For this review, take the finished solid that the model builds, in its own axes (mm). A direction names the side the tool comes from. Coordinates: 2 decimals unless noted, no trailing zeros. Loops run counter-clockwise (first coordinate to the right, second up) from the corner with the lowest first, then second, coordinate; pieces in that order, holes last. Notation, with made-up numbers: (20, 0.5) - (47, 0.5) arc R21 ccw to (47, 13.5) - close; hole circle Ø5 at (89, 19). An arc over 180 degrees is marked (long way). Use one line per item in the form item = value. Start each with the question number.
1. To check wall thickness, follow probe 1 along Y at (x, z) = (0, 12); probe 2 along X at (y, z) = (-37, 14); probe 3 along X at (y, z) = (9, 3.5). State the ranges of each line that lie inside material, in increasing order.
2. For pin 1 Ø1.2 at (x, y) = (-40, 1) entering from +Z; pin 2 Ø2.5 at (x, y) = (2.5, 40.5) entering from +Z; pin 3 Ø2 at (x, z) = (11, 13.5) entering from -Y; pin 4 Ø1 at (x, z) = (39.5, 3) entering from -Y, all flat-tipped, find the tip position at first contact; note any pin that passes through.
3. Draft analysis for pull direction X (two halves, no side actions). For faces 1 (the face through (40, 5, 2)), 2 (the face through (-10, -40, 16.7)), 3 (the face through (20.765, 39.923, 8.233)), state which applies: +X half, -X half, draft (parallel to the pull), parting line (faces both ways), or undercut.
4. Machinability: for faces 4 (the face through (0, 40, 4)), 5 (the face through (-40, 0, 0)), 6 (the face through (39, 0, 2)), which of the approach directions +Z, -Z, +X, -X, +Y, -Y give a long, thin tool a straight path to every point of the face, cutting with its end or side? Answer none if there is none.
5. Add section A-A on y = 0. Give the boundary of the cut face in (x, z), and give its area (3 significant figures).
6. Add section C-C on z = 7. Give the boundary of the cut face in (x, y).
7. Add section D-D on x = 26.5. Give the boundary of the cut face in (y, z), and give its area (3 significant figures).
Autodesk Inventor part; units mm, degrees
ref_plane "YZ Plane" through (0, 0, 0) normal (1, 0, 0) x (0, 1, 0)
ref_plane "XZ Plane" through (0, 0, 0) normal (0, 1, 0) x (-1, 0, 0)
ref_plane "XY Plane" through (0, 0, 0) normal (0, 0, 1) x (1, 0, 0)
sketch "Sketch1" plane through (0, 0, 0) normal (0, 0, 1) x (1, 0, 0)
  circle A0 centre (0, 0) radius 16.5
  circle A1 centre (0, 0) radius 22
  circle A2 centre (0, 0) radius 41
  circle A3 centre (0, 0) radius 45
  line L0 (0, 0) -> (-82.1679, 0) construction
  line L1 (0, 0) -> (52.3587, 0) construction
  line L2 (0, 0) -> (0, 55.2671) construction
  line L3 (0, 0) -> (0, -51.5979) construction
  circle A4 centre (0, 0) radius 39
  line L4 (5, 40.694) -> (5, 38.6782)
  line L5 (-5, 40.694) -> (-5, 38.6782)
  arc A5 (5, 40.694) -> (-5, 40.694) centre (0, 0) ccw
  arc A6 (5, 38.6782) -> (-5, 38.6782) centre (0, 0) ccw
  dimension "d2" = 82
  dimension "d15" = 78
  dimension "d0" = 33
  dimension "d1" = 44
  dimension "d3" = 90
  dimension "d16" = 5
extrude "outer" add sketch "Sketch1" along normal blind 16.7 contours A3
extrude "inner" [suppressed]
extrude "Extrusion4" add sketch "Sketch1" along normal blind 4 contours L4 A4 L5 A2 picked at (3.8902, 39.4454)
pattern_circular "Circular Pattern1" count 4 over 360 about axis through (0, 0, -10) along (0, 0, 1) of "Extrusion4"
equation "\"d15\" = PCB_OD"
equation "\"d0\" = skeleton_OD"
equation "\"d1\" = PCB_ID"
equation "\"d3\" = carbon_OD"
equation "\"PCB_OD\" = 78"
equation "\"PCB_ID\" = 44"
equation "\"skeleton_OD\" = 33"
equation "\"carbon_OD\" = 90"
properties part number "hall_case"
Conclusion:
q1.probe_1 = -45 to -41, 41 to 45
q1.probe_2 = -25.61 to -17.66, 17.66 to 25.61
q1.probe_3 = -44.09 to -40, 40 to 44.09
q2.pin_1 = 4
q2.pin_2 = 16.7
q2.pin_3 = -43.87
q2.pin_4 = -22.45
q3.face_1 = undercut
q3.face_2 = draft
q3.face_3 = parting line
q4.face_4 = +Z
q4.face_5 = -Z, +X, -X, +Y, -Y
q4.face_6 = +Z, -Z
q5.outline = (-45, 0) - (-39, 0) - (-39, 4) - (-41, 4) - (-41, 16.7) - (-45, 16.7) - close; (39, 0) - (45, 0) - (45, 16.7) - (41, 16.7) - (41, 4) - (39, 4) - close
q5.area = 150 mm^2
q6.outline = circle Ø90 at (0, 0); hole circle Ø82 at (0, 0)
q7.outline = (-36.37, 0) - (-31.28, 0) - (-31.28, 16.7) - (-36.37, 16.7) - close; (31.28, 0) - (36.37, 0) - (36.37, 16.7) - (31.28, 16.7) - close
q7.area = 170 mm^2
